```python
from build123d import *

# Parameters (mm, degrees)
SKETCH1_R           = 31.5
SKETCH1_R_2         = 22.625
BOSS_EXTRUDE1_DEPTH = 1.5
BOSS_EXTRUDE2_DEPTH = 5
CUT_EXTRUDE10_START = -4
CUT_EXTRUDE10_DEPTH = 4


# Read off the part's stored shape, not the designer's step: Cut-Extrude10
with BuildPart() as part:
    # Sketch1 → Boss-Extrude1 (new body)
    with BuildSketch(Plane(origin=(0, 0, 0), x_dir=(1, 0, 0), z_dir=(0, 1, 0))):
        with Locations(Location((0, 0, 0), (0, 0, 270))):
            Circle(SKETCH1_R)
        with Locations(Location((0, 0, 0), (0, 0, 270))):
            Circle(SKETCH1_R_2, mode=Mode.SUBTRACT)
        with BuildLine():
            ThreePointArc((-15.242434724, 21.37406298), (-12.068710047, 26.64067482), (-6.585582445, 29.423666069))
            ThreePointArc((-6.585582445, 29.423666069), (-4.653290128, 28.115519899), (-5.961436298, 26.183227582))
            ThreePointArc((-5.961436298, 26.183227582), (-9.821558376, 24.224001618), (-12.05586069, 20.516306647))
            ThreePointArc((-12.05586069, 20.516306647), (-14.078025873, 19.351897797), (-15.242434724, 21.37406298))
        make_face(mode=Mode.SUBTRACT)
        with BuildLine():
            ThreePointArc((15.786701292, 17.805692285), (20.00336614, 16.826485265), (23.059544082, 13.760725128))
            ThreePointArc((23.059544082, 13.760725128), (25.301502679, 13.113715353), (25.948512455, 15.35567395))
            ThreePointArc((25.948512455, 15.35567395), (21.607350881, 19.710446595), (15.617770512, 21.101365568))
            ThreePointArc((15.617770512, 21.101365568), (14.05439926, 19.369063536), (15.786701292, 17.805692285))
        make_face(mode=Mode.SUBTRACT)
        with BuildLine():
            ThreePointArc((21.812578659, -9.511783622), (22.18431854, -13.824661813), (20.213018306, -17.678631743))
            ThreePointArc((20.213018306, -17.678631743), (20.29047875, -20.010798092), (22.622645099, -19.933337648))
            ThreePointArc((22.622645099, -19.933337648), (25.422787299, -14.458948891), (24.894747729, -8.33270185))
            ThreePointArc((24.894747729, -8.33270185), (22.764122308, -7.381158201), (21.812578659, -9.511783622))
        make_face(mode=Mode.SUBTRACT)
        with BuildLine():
            ThreePointArc((-2.305786299, -23.684297857), (-6.292703266, -25.370596148), (-10.567211754, -24.68672042))
            ThreePointArc((-10.567211754, -24.68672042), (-12.761297164, -25.481068715), (-11.966948868, -27.675154125))
            ThreePointArc((-11.966948868, -27.675154125), (-5.895204242, -28.646568451), (-0.231970274, -26.251258529))
            ThreePointArc((-0.231970274, -26.251258529), (0.01460205, -23.930870181), (-2.305786299, -23.684297857))
        make_face(mode=Mode.SUBTRACT)
        with BuildLine():
            ThreePointArc((-23.237632962, -5.125917453), (-26.073423039, -1.855228921), (-26.743914336, 2.421399453))
            ThreePointArc((-26.743914336, 2.421399453), (-28.177394138, 4.262631556), (-30.018626241, 2.829151754))
            ThreePointArc((-30.018626241, 2.829151754), (-29.066223891, -3.245604073), (-25.038113242, -7.891468169))
            ThreePointArc((-25.038113242, -7.891468169), (-22.755097744, -7.408932951), (-23.237632962, -5.125917453))
        make_face(mode=Mode.SUBTRACT)
    extrude(amount=BOSS_EXTRUDE1_DEPTH)

    # Sketch2 → Boss-Extrude2 (add)
    with BuildSketch(Plane(origin=(0, 1.5, 0), x_dir=(1, 0, 0), z_dir=(0, 1, 0))):
        with BuildLine():
            Line((-4.111485424, -29.212081193), (-4.390230198, -31.192561274))
            ThreePointArc((-4.390230198, -31.192561274), (7.554963543, -30.580590672), (18.410886017, -25.559524175))
            Line((18.410886017, -25.559524175), (17.241940873, -23.936697244))
            ThreePointArc((17.241940873, -23.936697244), (7.075283318, -28.638965868), (-4.111485424, -29.212081193))
        make_face()
    extrude(amount=BOSS_EXTRUDE2_DEPTH)

    # Cut-Extrude10 outline → Cut-Extrude10 (cut)
    with BuildSketch(Plane(origin=(0, 6.5, 0), x_dir=(1, 0, 0), z_dir=(0, 1, 0)).offset(CUT_EXTRUDE10_START)):
        with BuildLine():
            Line((16.588514576, -24.394080925), (16.588514576, -26.778184855))
            ThreePointArc((16.588514576, -26.778184855), (17.510305364, -26.184713213), (18.410886017, -25.559524175))
            Line((18.410886017, -25.559524175), (17.241940873, -23.936697244))
            ThreePointArc((17.241940873, -23.936697244), (16.916773597, -24.167597545), (16.588514576, -24.394080925))
        make_face()
        with BuildLine():
            ThreePointArc((11.988514576, -29.129461345), (13.14913076, -28.624296677), (14.288514576, -28.072911342))
            Line((14.288514576, -28.072911342), (14.288514576, -25.808687515))
            ThreePointArc((14.288514576, -25.808687515), (13.150991563, -26.406465514), (11.988514576, -26.954137313))
            Line((11.988514576, -26.954137313), (11.988514576, -29.129461345))
        make_face()
        with BuildLine():
            ThreePointArc((7.388514576, -30.621232052), (8.544663351, -30.318949985), (9.688514576, -29.973032634))
            Line((9.688514576, -29.973032634), (9.688514576, -27.863644509))
            ThreePointArc((9.688514576, -27.863644509), (8.545605603, -28.235131041), (7.388514576, -28.559759319))
            Line((7.388514576, -28.559759319), (7.388514576, -30.621232052))
        make_face()
        with BuildLine():
            Line((-4.111485424, -29.212081193), (-4.390230198, -31.192561274))
            ThreePointArc((-4.390230198, -31.192561274), (-4.250900192, -31.211854279), (-4.111485424, -31.230524933))
            Line((-4.111485424, -31.230524933), (-4.111485424, -29.212081193))
        make_face()
        with BuildLine():
            ThreePointArc((2.788514576, -31.376331628), (3.941183712, -31.252473037), (5.088514576, -31.086283461))
            Line((5.088514576, -31.086283461), (5.088514576, -29.057822001))
            ThreePointArc((5.088514576, -29.057822001), (3.941565151, -29.235493226), (2.788514576, -29.367910829))
            Line((2.788514576, -29.367910829), (2.788514576, -31.376331628))
        make_face()
        with BuildLine():
            Line((-1.811485424, -29.444329175), (-1.811485424, -31.447869889))
            ThreePointArc((-1.811485424, -31.447869889), (-0.270009845, -31.498842752), (1.272113036, -31.474302668))
            Line((1.272113036, -31.474302668), (0.488514576, -31.474302668))
            Line((0.488514576, -31.474302668), (0.488514576, -29.495954867))
            ThreePointArc((0.488514576, -29.495954867), (-0.661988874, -29.49257145), (-1.811485424, -29.444329175))
        make_face()
    extrude(amount=CUT_EXTRUDE10_DEPTH, mode=Mode.SUBTRACT)


solid = part.part
```
The model under review builds one solid part; all positions refer to its coordinate system, in mm. A direction names the side the tool comes from. Round coordinates to 2 decimals unless told otherwise and drop trailing zeros. Order: outer loops, then holes, each group sorted by start corner. A loop starts at its lowest first (then second) coordinate and runs counter-clockwise, first axis right, second up.
(1) Take a section at C-C, the plane x = 6. State the section outline as (y, z) points, plus the area to 3 significant figures.
Working result:
outline: (0, -30.92) - (1.5, -30.92) - (1.5, -21.81) - (0, -21.81) - close; (0, 21.81) - (1.5, 21.81) - (1.5, 28.88) - (6.5, 28.88) - (6.5, 30.92) - (0, 30.92) - close
area: 37.5 mm2
(2) Take a section at A-A, the plane z = -8. State the section outline as (x, y) points.
Working result:
outline: (-30.47, 0) - (-21.16, 0) - (-21.16, 1.5) - (-30.47, 1.5) - close; (21.16, 0) - (30.47, 0) - (30.47, 1.5) - (21.16, 1.5) - close
(3) Wall thickness on L1, parallel to X at y = 0.7, z = 0 (3 decimals); L2, parallel to Y at x = 25.5, z = -16.5: over which ranges is each line inside the solid? List them lowest first.
Working result:
L1: x = -31.5 to -30.009, -26.669 to -22.625, 22.625 to 31.5
L2: y = 0 to 1.5
(4) Mouldability with a two-part tool opening along X and no side actions: class faces 4 (the face through (-4.111, 4, 30)), 5 (the face through (6, 6.5, 30)), 6 (the face through (0.489, 4, 30)) as released by +X, released by -X, zero draft, split by the parting line, or undercut.
Working result:
face 4: released by -X
face 5: zero draft
face 6: undercut
(5) For P1, Ø0.6, axis at y = 4.5, z = 29.5, coming from the +X side; P2, Ø0.6, axis at y = 4, z = 30.5, coming from the +X side; P3, Ø1.8, axis at x = 4, z = 30, coming from the +Y side, all flat-tipped, find the tip position at first contact; note any pin that passes through.
Working result:
P1: stops at x = 11.82
P2: stops at x = 7.39
P3: stops at y = 2.5
(6) Take a section at D-D, the plane z = 0. State the section outline as (x, y) points (3 decimals).
Working result:
outline: (-31.5, 0) - (-30.009, 0) - (-30.009, 1.5) - (-31.5, 1.5) - close; (-26.669, 0) - (-22.625, 0) - (-22.625, 1.5) - (-26.669, 1.5) - close; (22.625, 0) - (31.5, 0) - (31.5, 1.5) - (22.625, 1.5) - close
(7) Tool access review of faces 1 (the face through (14.053, 0.74, -19.405)), 2 (the face through (7.23, 3.41, 28.6)), 3 (the face through (2.789, 4, 30)): name each direction out of +Z, -Z, +X, -X, +Y, -Y from which nothing blocks a thin tool from reaching the whole face with its end or side.
Working result:
face 1: +Y, -Y
face 2: -Z, +Y
face 3: +Z, -Z, +Y
(8) Take a section at B-B, the plane y = 3.25. State the section outline as (x, z) points.
Working result:
outline: (-4.11, 29.21) arc R29.5 cw to (-1.81, 29.44) - (-1.81, 31.45) arc R31.5 ccw to (-4.11, 31.23) - close; (0.49, 29.5) arc R29.5 cw to (2.79, 29.37) - (2.79, 31.38) arc R31.5 ccw to (1.27, 31.47) - (0.49, 31.47) - close; (5.09, 29.06) arc R29.5 cw to (7.39, 28.56) - (7.39, 30.62) arc R31.5 ccw to (5.09, 31.09) - close; (9.69, 27.86) arc R29.5 cw to (11.99, 26.95) - (11.99, 29.13) arc R31.5 ccw to (9.69, 29.97) - close; (14.29, 25.81) arc R29.5 cw to (16.59, 24.39) - (16.59, 26.78) arc R31.5 ccw to (14.29, 28.07) - close
